Source: CAD feature listing. Evaluate the final solid. Frame: model axes, mm. Face numbers are marked on the shaded views. A direction names the side the tool comes from. Give positions to 0.01 mm unless a question says otherwise; leave off trailing zeros. Order: outer loops, then holes, each group sorted by start corner. A loop starts at its lowest first (then second) coordinate and runs counter-clockwise, first axis right, second up. Notation, with made-up numbers: M -19.5,43 L -9.5,43 A26 ccw -9.5,65 Z; hole C -17,-12.5 d2. An arc over 180 degrees is marked long. Return JSON: item names as keys, results as strings.
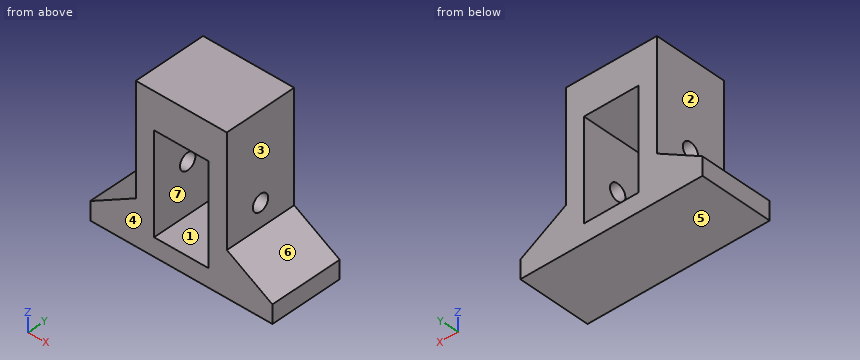
from build123d import *

# Parameters (mm, degrees)
F0_W      = 50
F0_H      = 20
F1_DEPTH  = 5
F2_W      = 17.5
F2_H      = 20
F3_DEPTH  = 20
F5_DEPTH  = 20.001
F6_R      = 2.286
F7_DEPTH  = 37.501
F8_DEPTH  = 17.35
F9_W      = 20
F9_H      = 10
F10_DEPTH = 25


with BuildPart() as f1:
    # F0 (on Top) → F1 (new body)
    with BuildSketch(Plane.XY):
        Rectangle(F0_W, F0_H)
    extrude(amount=F1_DEPTH)

    # F2 (on face) → F3 (join)
    with BuildSketch(Plane.XY.offset(5)):
        with Locations((16.25, 0)):
            Rectangle(F2_W, F2_H)
        with Locations((-16.25, 0)):
            Rectangle(F2_W, F2_H)
    extrude(amount=F3_DEPTH)

    # F4 (on face) → F5 (cut, through all)
    with BuildSketch(Plane(origin=(0, 10, 0), x_dir=(-1, 0, 0), z_dir=(0, 1, 0))):
        Polygon((-25, 5), (-12.5, 12.3), (-12.5, 25), (-25, 25), align=None)
        Polygon((12.5, 25), (12.5, 12.3), (25, 5), (25, 25), align=None)
    extrude(amount=-F5_DEPTH, mode=Mode.SUBTRACT)

    # F6 (on face) → F7 (cut, through all)
    with BuildSketch(Plane(origin=(-12.5, 0, 0), x_dir=(0, -1, 0), z_dir=(-1, 0, 0))):
        with Locations((0, 18.65)):
            Circle(F6_R)
    extrude(amount=-F7_DEPTH, mode=Mode.SUBTRACT)

    # F8 (add): faces of the model
    f8_faces = [f1.faces().sort_by_distance(p)[0] for p in [
        (-10, 0, 25),
        (10, 0, 25),
    ]]
    extrude(f8_faces, amount=F8_DEPTH)

    # F9 (on face) → F10 (join, through all)
    with BuildSketch(Plane.YZ.offset(12.5)):
        with Locations((0, 37.35)):
            Rectangle(F9_W, F9_H)
    extrude(amount=-F10_DEPTH)


solid = f1.part
1. Ray query, probe 1 along X at (y, z) = (-2.5, 31); probe 2 along Z at (x, y) = (11.3, 0); probe 3 along Z at (x, y) = (3, 3.25). Return the intervals inside material, ascending.
Evaluation:
{"probe 1": "x = -12.5 to -7.5, 7.5 to 12.5", "probe 2": "z = 0 to 16.36, 20.94 to 42.35", "probe 3": "z = 0 to 5, 32.35 to 42.35"}
2. Section query C-C (x = 2). Return loops of the section in (y, z), then the cut area to 3 significant figures.
Evaluation:
{"outline": "M -10,0 L 10,0 L 10,5 L -10,5 Z; M -10,32.35 L 10,32.35 L 10,42.35 L -10,42.35 Z", "area": "300 mm^2"}
3. Section query D-D (y = 0). Return loops of the section in (x, z), then the cut area to 3 significant figures.
Evaluation:
{"outline": "M -25,0 L 25,0 L 25,5 L 12.5,12.3 L 12.5,16.36 L 7.5,16.36 L 7.5,5 L -7.5,5 L -7.5,16.36 L -12.5,16.36 L -12.5,12.3 L -25,5 Z; M -12.5,20.94 L -7.5,20.94 L -7.5,32.35 L 7.5,32.35 L 7.5,20.94 L 12.5,20.94 L 12.5,42.35 L -12.5,42.35 Z", "area": "819 mm^2"}
4. Set-up query: the marked faces 1, 2 and 3. Return all of +Z, -Z, +X, -X, +Y, -Y with unobstructed straight access to the full face (end or side cutting, diameter ignored); none if empty.
Evaluation:
{"face 1": "+Y, -Y", "face 2": "+Z, -X, +Y, -Y", "face 3": "+Z, +X, +Y, -Y"}
5. Section query B-B (y = 7.5). Return loops of the section in (x, z).
Evaluation:
{"outline": "M -25,0 L 25,0 L 25,5 L 12.5,12.3 L 12.5,42.35 L -12.5,42.35 L -12.5,12.3 L -25,5 Z; hole M -7.5,5 L 7.5,5 L 7.5,32.35 L -7.5,32.35 Z"}
6. Draft query along Z for the marked faces 4, 5, 6 and 7. Return one class per face: pulls with the +Z half, pulls with the -Z half, needs draft (parallel to the pull), parting line crosses it, or undercut.
Evaluation:
{"face 4": "needs draft", "face 5": "pulls with the -Z half", "face 6": "pulls with the +Z half", "face 7": "undercut"}
7. First-contact query: pin 1 (6 mm diameter, centred on y = -3, z = 31.5, fed in from +X); pin 2 (1 mm diameter, centred on y = 6, z = 29.5, fed in from -X); pin 3 (7.5 mm diameter, centred on x = -2, y = -2.5, fed in from -Z). Flat tips, straight axial feed; report the tip coordinate or a pass-through.
Evaluation:
{"pin 1": "stops at x = 12.5", "pin 2": "stops at x = -12.5", "pin 3": "stops at z = 0"}
8. Section query A-A (z = 13.5). Return loops of the section in (x, y), then the cut area to 3 significant figures.
Evaluation:
{"outline": "M -12.5,-10 L -7.5,-10 L -7.5,10 L -12.5,10 Z; M 7.5,-10 L 12.5,-10 L 12.5,10 L 7.5,10 Z", "area": "200 mm^2"}
